from build123d import *

# Parameters (mm, degrees)
SKETCH4_R             = 1.5
CUT_EXTRUDE1_DEPTH    = 85.285208987
CUT_LOFT1_START       = -30.432295628
CUT_LOFT1_DEPTH       = 40.932295728
CUT_LOFT1_START_2     = -9.276423483
CUT_LOFT1_2_DEPTH     = 37.189014281
CUT_LOFT1_START_3     = -30
CUT_LOFT1_3_OUTLINE_W = 25.432295628
CUT_LOFT1_3_OUTLINE_H = 72
CUT_LOFT1_3_DEPTH     = 19.959259101
CUT_LOFT1_START_4     = 10.040740899
CUT_LOFT1_4_OUTLINE_W = 25.432295628
CUT_LOFT1_4_OUTLINE_H = 72
CUT_LOFT1_4_DEPTH     = 16.959259101
SKETCH10_R            = 2.5
CUT_EXTRUDE2_DEPTH    = 10
SKETCH11_R            = 2.5
CUT_EXTRUDE3_DEPTH    = 10
BOSS_EXTRUDE1_DEPTH   = 4.8
SKETCH14_W            = 37.12113751
SKETCH14_H            = 26.161757616
CUT_EXTRUDE4_DEPTH    = 3
SKETCH15_W            = 15.761114721
SKETCH15_H            = 46.929857457
CUT_EXTRUDE5_DEPTH    = 3


with BuildPart() as part:
    # Loft1: read off the stored shape, not the designer's step
    # Loft1: loft between two sections, ruled curve by curve
    loft1_from = [
        Edge.make_line((-34.432295528, 31.912590798, 70), (-34.432295528, 10.912590798, 70)),
        Edge.make_line((-34.432295528, 10.912590798, 70), (-13.432295528, 10.912590798, 70)),
        Edge.make_line((-13.432295528, 10.912590798, 70), (-13.432295528, 31.912590798, 70)),
        Edge.make_line((-13.432295528, 31.912590798, 70), (-34.432295528, 31.912590798, 70)),
    ]
    loft1_to = [
        Edge.make_line((-10.5, 10.5, 0), (-10.5, -10.5, 0)),
        Edge.make_line((-10.5, -10.5, 0), (10.5, -10.5, 0)),
        Edge.make_line((10.5, -10.5, 0), (10.5, 10.5, 0)),
        Edge.make_line((10.5, 10.5, 0), (-10.5, 10.5, 0)),
    ]
    loft1 = Solid(Shell([*[Face.make_surface_from_curves(loft1_from[k], loft1_to[k]) for k in range(4)], Face(Wire(loft1_from)), Face(Wire(loft1_to))]))
    add(loft1)

    # Sketch4 → Cut-Extrude1 (cut, through all)
    with BuildSketch(Plane(origin=(0, 0, 0), x_dir=(-1, 0, 0), z_dir=(0, 0, -1))):
        with Locations((3.5, -5.5)):
            Circle(SKETCH4_R)
        with Locations((-5.5, -5.5)):
            Circle(SKETCH4_R)
        with Locations((-5.5, 3.5)):
            Circle(SKETCH4_R)
        with Locations((3.5, 3.5)):
            Circle(SKETCH4_R)
    extrude(amount=-CUT_EXTRUDE1_DEPTH, mode=Mode.SUBTRACT)

    # Cut-Loft1: read off the stored shape, not the designer's step
    # Cut-Loft1 outline → Cut-Loft1 (cut)
    with BuildSketch(Plane.YZ.offset(CUT_LOFT1_START)):
        Polygon((10.912590798, 70), (-9.276423383, 4), (6.5, 4), (27.912590798, 70), align=None)
    extrude(amount=CUT_LOFT1_DEPTH, mode=Mode.SUBTRACT)

    # Cut-Loft1 2 outline → Cut-Loft1 2 (add)
    with BuildSketch(Plane(origin=(0, 0, 0), x_dir=(1, 0, 0), z_dir=(0, 1, 0)).offset(CUT_LOFT1_START_2)):
        Polygon((-6.5, -4), (-11.867559744, -4), (-30.432295628, -58.300328622), (-30.432295628, -70), align=None)
    extrude(amount=CUT_LOFT1_2_DEPTH)

    # Cut-Loft1 3 outline → Cut-Loft1 3 (cut)
    with BuildSketch(Plane(origin=(0, 0, 0), x_dir=(1, 0, 0), z_dir=(0, 0.9562610380135655, -0.2925146614739479)).offset(CUT_LOFT1_START_3)):
        with Locations((-17.716147814, -36)):
            Rectangle(CUT_LOFT1_3_OUTLINE_W, CUT_LOFT1_3_OUTLINE_H)
    extrude(amount=CUT_LOFT1_3_DEPTH, mode=Mode.SUBTRACT)

    # Cut-Loft1 4 outline → Cut-Loft1 4 (cut)
    with BuildSketch(Plane(origin=(0, 0, 0), x_dir=(1, 0, 0), z_dir=(0, 0.9562610380135655, -0.2925146614739479)).offset(CUT_LOFT1_START_4)):
        with Locations((-17.716147814, -36)):
            Rectangle(CUT_LOFT1_4_OUTLINE_W, CUT_LOFT1_4_OUTLINE_H)
    extrude(amount=CUT_LOFT1_4_DEPTH, mode=Mode.SUBTRACT)

    # Sketch10 → Cut-Extrude2 (cut)
    with BuildSketch(Plane(origin=(0, 9.601569315, -2.937063925), x_dir=(1, 0, 0), z_dir=(0, 0.9562610380135655, -0.29251466147394767))):
        with Locations(Location((-4.504228797, -16.617876366, 0), (0, 0, 270))):
            Circle(SKETCH10_R)
    extrude(amount=-CUT_EXTRUDE2_DEPTH, mode=Mode.SUBTRACT)

    # Sketch11 → Cut-Extrude3 (cut)
    with BuildSketch(Plane(origin=(-9.401115557, 0, -3.214146797), x_dir=(-0.3235052723680801, 0, 0.9462263676045255), z_dir=(-0.9462263676045255, 0, -0.3235052723680801))):
        with Locations((18.022307071, 3.324420334)):
            Circle(SKETCH11_R)
    extrude(amount=-CUT_EXTRUDE3_DEPTH, mode=Mode.SUBTRACT)

    # Sketch13 → Boss-Extrude1 (add)
    with BuildSketch(Plane(origin=(0, 0, 0), x_dir=(-1, 0, 0), z_dir=(0, 0, -1))):
        Polygon((10.5, -10.5), (10.5, 10.5), (-10.5, 10.5), (-10.5, 7.5), (7.5, 7.5), (7.5, -10.5), align=None)
    extrude(amount=BOSS_EXTRUDE1_DEPTH)

    # Sketch14 → Cut-Extrude4 (cut)
    with BuildSketch(Plane(origin=(0, 9.601569315, -2.937063925), x_dir=(1, 0, 0), z_dir=(0, 0.9562610380135657, -0.2925146614739477))):
        with Locations((-1.808901269, 4.696953713)):
            Rectangle(SKETCH14_W, SKETCH14_H)
    extrude(amount=CUT_EXTRUDE4_DEPTH, mode=Mode.SUBTRACT)

    # Sketch15 → Cut-Extrude5 (cut)
    with BuildSketch(Plane(origin=(-9.401115557, 0, -3.214146797), x_dir=(-0.32350527236808013, 0, 0.9462263676045254), z_dir=(-0.9462263676045255, 0, -0.32350527236808013))):
        with Locations((3.08021958, -4.471111323)):
            Rectangle(SKETCH15_W, SKETCH15_H)
    extrude(amount=CUT_EXTRUDE5_DEPTH, mode=Mode.SUBTRACT)


solid = part.part
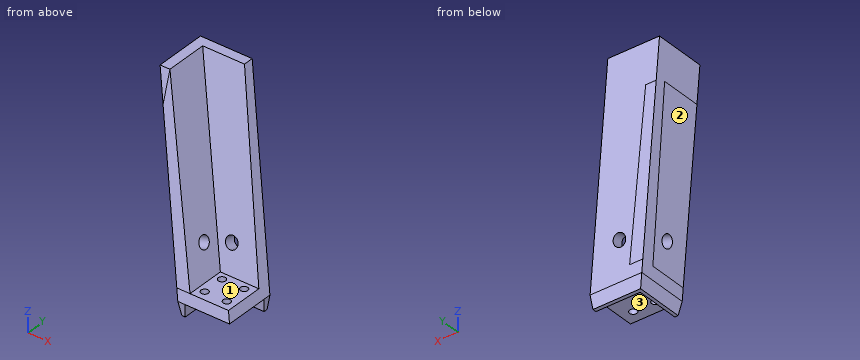
Can you work these out from the model? Positions are in its coordinate system, mm. Face numbers are marked on the shaded views. A direction names the side the tool comes from. Give positions to 0.01 mm unless a question says otherwise; leave off trailing zeros. Answer as a JSON object with one key per item and string values.
Q1. If I drill on L1, parallel to Y at x = 5.5, z = 3.1; L2, parallel to Y at x = -3.5, z = 2.7; L3, parallel to Z at x = -1.5, y = 5, over which ranges is the centre line in solid material (lowest first)?
Geometry says:
{"L1": "-9.55 to -7, -4 to 2, 5 to 11.45", "L2": "-9.67 to -7, -4 to 2, 5 to 11.33", "L3": "0 to 4"}
Q2. Imagine slicing it at A-A on y = -5.5. Give the number of separate pieces and of enclosed holes in the cut face, plus the area to 3 significant figures.
Geometry says:
{"separate pieces": "3", "enclosed holes": "0", "area": "135 mm²"}
Q3. Which directions (+Z, -Z, +X, -X, +Y, -Y) give clear straight access to the entire face, cutting with the end or side of a thin tool? Please do the marked faces 1, 2 and 3.
Geometry says:
{"face 1": "+Z, +X, -Y", "face 2": "-Z, -X, +Y, -Y", "face 3": "-Z, +X, -Y"}
Q4. Will these pins go through, and if not, where does the flat tip stop? P1, Ø8, axis at x = -19.5, z = 11.5, coming from the -Y side; P2, Ø3.5, axis at x = -3.5, y = -5.5, coming from the -Z side; P3, Ø8, axis at x = -3.5, z = 49.5, coming from the -Y side; P4, Ø12, axis at y = 14, z = 50, coming from the +X side.
Geometry says:
{"P1": "through", "P2": "z = 0", "P3": "y = 20.08", "P4": "x = -21"}
